The listing builds one solid part. Answer for the finished solid, in the listing's coordinates (mm). A direction names the side the tool comes from. Coordinates: 2 decimals unless noted, no trailing zeros. Order: outer loops, then holes, each group sorted by start corner. A loop starts at its lowest first (then second) coordinate and runs counter-clockwise, first axis right, second up. Notation, with made-up numbers: (48, 24.5) - (71, 24.5) arc R23 ccw to (71, 50.5) - close; hole circle Ø7 at (18, 0.5). An arc over 180 degrees is marked (long way). Use a Markdown table: item, result. Add a question column.
Item 1: The mould has two halves that part along Z. Classify faces 1 (the flat face through (-45, 130.4, -26.6)), 2 (the cylindrical face through (44.01, 7.81, -1.73)), 3 (the cylindrical face through (43.99, 4.46, 0.59)): released by +Z, released by -Z, zero draft, split by the parting line, or undercut.
Item 2: The part is cut by section A-A, the plane x = 19.5. Give the vertices of the cut face in (y, z), then the cut area to 3 significant figures.
Item 3: Find the intervals of material crossed by line 1 along Y through (x, z) = (-36, -159); line 2 along X through (y, z) = (12, 2.5); line 3 along Y through (x, z) = (-27.5, -157), in increasing order.
Item 4: For faces 4 (the flat face through (45, 3.4, 3.4)), 5 (the cylindrical face through (-8.165, 154.706, -158.124)), 6 (the cylindrical face through (44, 134.8, -31.8)), determine the directions among +Z, -Z, +X, -X, +Y, -Y from which every point of the face is accessible in a straight line to the end or side of a thin tool.
Item 5: The part is cut by section C-C, the plane z = -107.5. Give the vertices of the cut face in (x, y), then the cut area to 3 significant figures.
Item 6: Flat-ended cylindrical pins translate along their axes: P1, Ø4.5, axis at y = 159.5, z = -159.5, coming from the +X side; P2, Ø5, axis at y = 4, z = 3.5, coming from the -X side; P3, Ø11.5, axis at y = 152.74, z = -119.94, coming from the -X side. Find the tip coordinate at first contact, or state that the pin passes through.
Item 7: The part is cut by section B-B, the plane y = 110.5. Give the vertices of the cut face in (x, z), then the cut area to 3 significant figures.
from build123d import *

# Parameters (mm, degrees)
SKETCH1_R                   = 8
MOUNT_TUBES_DEPTH           = 45
MOUNT_TUBES_2_DEPTH         = 45
MOUNT_TUBES_3_DEPTH         = 45
SKETCH2_R                   = 8
EXTEND_TUBE_1_DEPTH         = 10
MOUNT_TUBE_HOLES_DEPTH      = 243.629694853
MOUNT_TUBE_HOLES_DEPTH_BACK = 243.629694853
SKETCH3_R                   = 4.5
SIDE_PLATE_RH_DEPTH         = 3
MOTOR_MOUNT_HOLES_R         = 5
MOTOR_MOUNT_HOLES_F_DEPTH   = 247.763767871


with BuildPart() as part:
    # Sketch1 → mount tubes (new, symmetric)
    with BuildSketch(Plane(origin=(0, 0, 0), x_dir=(0, 0, -1), z_dir=(1, 0, 0))):
        with Locations(Location((0, 0, 0), (0, 0, 180))):
            Circle(SKETCH1_R)
    extrude(amount=MOUNT_TUBES_DEPTH, both=True)


with BuildPart() as body_2:
    # Sketch1 → mount tubes 2 (new, symmetric)
    with BuildSketch(Plane(origin=(0, 0, 0), x_dir=(0, 0, -1), z_dir=(1, 0, 0))):
        with Locations(Location((30.031235259, 126.997538987, 0), (0, 0, 180))):
            Circle(SKETCH1_R)
    extrude(amount=MOUNT_TUBES_2_DEPTH, both=True)


with BuildPart() as body_3:
    # Sketch1 → mount tubes 3 (new, symmetric)
    with BuildSketch(Plane(origin=(0, 0, 0), x_dir=(0, 0, -1), z_dir=(1, 0, 0))):
        with Locations(Location((159.099025767, 159.099025767, 0), (0, 0, 180))):
            Circle(SKETCH1_R)
    extrude(amount=MOUNT_TUBES_3_DEPTH, both=True)

    # Sketch2 → extend tube 1 (add)
    with BuildSketch(Plane.ZY.offset(45)):
        with Locations((-159.099025767, 159.099025767)):
            Circle(SKETCH2_R)
    extrude(amount=EXTEND_TUBE_1_DEPTH)


with BuildPart() as mount_tube_holes_tool:
    # Sketch3 → mount tube holes (new, two sides: drawn at the far end of the back side and taken through both)
    with BuildSketch(Plane(origin=(0, 0, 0), x_dir=(0, 0, -1), z_dir=(1, 0, 0)).offset(-MOUNT_TUBE_HOLES_DEPTH_BACK)):
        Circle(SKETCH3_R)
        with Locations((30.031235259, 126.997538987)):
            Circle(SKETCH3_R)
        with Locations((159.099025767, 159.099025767)):
            Circle(SKETCH3_R)
    extrude(amount=MOUNT_TUBE_HOLES_DEPTH + MOUNT_TUBE_HOLES_DEPTH_BACK)


with BuildPart() as part_1:
    add(part.part)

    # mount tube holes: cut by mount_tube_holes_tool
    add(mount_tube_holes_tool.part, mode=Mode.SUBTRACT)



with BuildPart() as body_2_1:
    add(body_2.part)

    # mount tube holes: cut by mount_tube_holes_tool
    add(mount_tube_holes_tool.part, mode=Mode.SUBTRACT)


with BuildPart() as body_3_1:
    add(body_3.part)

    # mount tube holes: cut by mount_tube_holes_tool
    add(mount_tube_holes_tool.part, mode=Mode.SUBTRACT)


with BuildPart() as part_2:
    add(part_1.part)

    add(body_2_1.part)  # Side plate RH merges body 2

    add(body_3_1.part)  # Side plate RH merges body 3
    # Sketch4 → Side plate RH (add)
    with BuildSketch(Plane(origin=(40, 0, 0), x_dir=(0, 0, -1), z_dir=(1, 0, 0))):
        with BuildLine():
            Line((12.978386159, -0.749328179), (16.807561824, 65.572107296))
            ThreePointArc((16.807561824, 65.572107296), (23.501336664, 93.821843391), (39.475404328, 118.064025087))
            ThreePointArc((39.475404328, 118.064025087), (41.072624736, 120.135489845), (42.222827025, 122.484769304))
            ThreePointArc((42.222827025, 122.484769304), (54.40469235, 135.330973688), (72.108350397, 135.388433283))
            ThreePointArc((72.108350397, 135.388433283), (74.814895184, 134.666747236), (77.615418999, 134.724034171))
            Line((77.615418999, 134.724034171), (160.862063178, 148.241231374))
            ThreePointArc((160.862063178, 148.241231374), (169.95682016, 160.862063178), (157.335988356, 169.95682016))
            Line((157.335988356, 169.95682016), (74.089344178, 156.439622958))
            ThreePointArc((74.089344178, 156.439622958), (45.006724073, 152.267651322), (20.587066191, 135.931052888))
            ThreePointArc((20.587066191, 135.931052888), (-0.368139217, 104.129516319), (-9.149210493, 67.070763654))
            Line((-9.149210493, 67.070763654), (-9.268320599, 65.007773101))
            ThreePointArc((-9.268320599, 65.007773101), (-8.774360407, 63.178125859), (-7.282312147, 62.009623531))
            ThreePointArc((-7.282312147, 62.009623531), (3.971735746, 45.020109305), (-9.16284655, 29.438712206))
            ThreePointArc((-9.16284655, 29.438712206), (-10.779462777, 28.449693665), (-11.480714014, 26.689053894))
            Line((-11.480714014, 26.689053894), (-12.978386159, 0.749328179))
            ThreePointArc((-12.978386159, 0.749328179), (-0.749328179, -12.978386159), (12.978386159, -0.749328179))
        make_face()
    extrude(amount=SIDE_PLATE_RH_DEPTH)

    # motor mount holes → motor mount holes f (cut, through all)
    with BuildSketch(Plane(origin=(0, 0, 0), x_dir=(0, 0, -1), z_dir=(1, 0, 0))):
        with Locations(Location((119.938657263, 152.740349945, 0), (0, 0, 180))):
            Circle(MOTOR_MOUNT_HOLES_R)
        with Locations(Location((5.756211189, 65, 0), (0, 0, 180))):
            Circle(MOTOR_MOUNT_HOLES_R)
    extrude(amount=MOTOR_MOUNT_HOLES_F_DEPTH, mode=Mode.SUBTRACT)


solid = part_2.part
Solution:
| question | item | result |
|---|---|---|
| 1 | face 1 | zero draft |
| 1 | face 2 | split by the parting line |
| 1 | face 3 | undercut |
| 2 | outline | circle Ø16 at (0, 0); circle Ø16 at (127, -30.03); circle Ø16 at (159.1, -159.1); hole circle Ø9 at (0, 0); hole circle Ø9 at (127, -30.03); hole circle Ø9 at (159.1, -159.1) |
| 2 | area | 412 mm2 |
| 3 | line 1 | y = 151.1 to 154.6, 163.6 to 167.1 |
| 3 | line 2 | x = 40 to 43 |
| 3 | line 3 | y = 151.38 to 155.12, 163.08 to 166.82 |
| 4 | face 4 | +Z, -Z, +X, +Y, -Y |
| 4 | face 5 | -X |
| 4 | face 6 | +X |
| 5 | outline | (40, 139.58) - (43, 139.58) - (43, 161.86) - (40, 161.86) - close |
| 5 | area | 66.9 mm2 |
| 6 | P1 | stops at x = 43 |
| 6 | P2 | stops at x = -45 |
| 6 | P3 | stops at x = 40 |
| 7 | outline | (40, -33.13) - (43, -33.13) - (43, -2.63) - (40, -2.63) - close |
| 7 | area | 91.5 mm2 |
